Part model, mm, in its own coordinate system. A direction names the side the tool comes from. Give positions to 0.01 mm unless a question says otherwise; leave off trailing zeros. Order: outer loops, then holes, each group sorted by start corner. A loop starts at its lowest first (then second) coordinate and runs counter-clockwise, first axis right, second up. Notation, with made-up numbers: M 36.25,-8 L 81.25,-8 A21 cw 81.25,11 Z; hole C 57,47.25 d8. An arc over 180 degrees is marked long. Return JSON: item names as keys, results as strings.
from build123d import *

# Parameters (mm, degrees)
F0_W   = 1.27
F0_H   = 1.27
F0_W_2 = 3.81
F0_H_2 = 3.5783256781


with BuildPart() as f1:
    # F0 (on Front) → F1 (revolve)
    with BuildSketch(Plane.XZ):
        with BuildLine():
            Line((-12.7, 0), (0, 0))
            add(Edge.make_bspline(
                [(0, 0), (7.4514020234, 3.331559943), (-2.5339151704, 7.6260847131), (-2.54, 12.7)],
                knots=[0, 0, 0, 0, 12.9515095645, 12.9515095645, 12.9515095645, 12.9515095645], degree=3))
            Line((-2.54, 12.7), (-12.7, 12.7))
            Line((-12.7, 12.7), (-12.7, 0))
        make_face()
        with BuildLine():
            Line((-12.7, 12.7), (-2.54, 12.7))
            add(Edge.make_bspline(
                [(-2.54, 12.7), (4.5093661174, 26.4475625008), (-14.613872394, 38.6360026896), (-5.08, 50.8)],
                knots=[0, 0, 0, 0, 38.1845728011, 38.1845728011, 38.1845728011, 38.1845728011], degree=3))
            Line((-5.08, 50.8), (-12.7, 50.8))
            Line((-12.7, 50.8), (-12.7, 12.7))
        make_face()
        with BuildLine():
            Line((-12.7, 50.8), (-5.08, 50.8))
            add(Edge.make_bspline(
                [(-5.08, 50.8), (-3.208857961, 50.9595312178), (-3.3491132781, 53.203612566), (-5.08, 53.34)],
                knots=[0, 0, 0, 0, 2.54, 2.54, 2.54, 2.54], degree=3))
            Line((-5.08, 53.34), (-9.7673060372, 53.34))
            Line((-9.7673060372, 53.34), (-11.43, 53.34))
            Line((-11.43, 53.34), (-12.7, 53.34))
            Line((-12.7, 53.34), (-12.7, 50.8))
        make_face()
        with BuildLine():
            Line((-9.7673060372, 53.34), (-5.08, 53.34))
            Line((-5.08, 53.34), (-2.0844770548, 59.69))
            add(Edge.make_bspline(
                [(-11.43, 53.5471198024), (-8.0565585685, 54.6403665691), (-5.5479568491, 59.69), (-2.0844770548, 59.69)],
                knots=[1.3390316874, 1.3390316874, 1.3390316874, 1.3390316874, 12.3697949619, 12.3697949619, 12.3697949619, 12.3697949619], degree=3))
            Line((-11.43, 53.5471198024), (-11.43, 53.34))
            Line((-11.43, 53.34), (-9.7673060372, 53.34))
        make_face()
        with BuildLine():
            add(Edge.make_bspline(
                [(-12.7, 53.34), (-12.2617526092, 53.34), (-11.8395042981, 53.4144098506), (-11.43, 53.5471198024)],
                knots=[0, 0, 0, 0, 1.3390316874, 1.3390316874, 1.3390316874, 1.3390316874], degree=3))
            Line((-12.7, 53.34), (-11.43, 53.34))
            Line((-11.43, 53.34), (-11.43, 53.5471198024))
        make_face()
        with BuildLine():
            Line((-12.7, 61.1916743219), (-12.7, 53.34))
            add(Edge.make_bspline(
                [(-12.7, 53.34), (-12.2617526092, 53.34), (-11.8395042981, 53.4144098506), (-11.43, 53.5471198024)],
                knots=[0, 0, 0, 0, 1.3390316874, 1.3390316874, 1.3390316874, 1.3390316874], degree=3))
            Line((-11.43, 53.5471198024), (-11.43, 61.1916743219))
            Line((-11.43, 61.1916743219), (-12.7, 61.1916743219))
        make_face()
        with Locations((-12.065, 61.8266743219)):
            Rectangle(F0_W, F0_H)
        with Locations((-9.525, 61.8266743219)):
            Rectangle(F0_W_2, F0_H)
        with Locations((-12.065, 64.2508371609)):
            Rectangle(F0_W, F0_H_2)
    revolve(axis=Axis((-12.7, 0, 25.4), (0, 0, 1)))


with BuildPart() as f4:
    # F3 (on Front) → F4 (revolve)
    with BuildSketch(Plane.XZ):
        Polygon((-1.27, 83.82), (-1.7199835438, 78.9296406197), (0, 78.9296406197), (0, 83.82), align=None)
        Polygon((-4.4343151529, 77.1516406197), (-1.8835851687, 77.1516406197), (-1.7199835438, 78.9296406197), (-4.270713528, 78.9296406197), align=None)
        with BuildLine():
            Line((-15.5575, 0), (0, 0))
            Line((0, 0), (0, 55.88))
            Line((0, 55.88), (-5.08, 55.88))
            add(Edge.make_bspline(
                [(-15.5575, 7.62), (-12.4826701358, 22.7640494704), (-5.5103190243, 35.0550673902), (-5.08, 55.88)],
                knots=[0, 0, 0, 0, 49.3842647637, 49.3842647637, 49.3842647637, 49.3842647637], degree=3))
            Line((-15.5575, 7.62), (-15.5575, 5.08))
            ThreePointArc((-15.5575, 5.08), (-14.6594743879, 4.7080256121), (-14.2875, 3.81))
            ThreePointArc((-14.2875, 3.81), (-14.6594743879, 2.9119743879), (-15.5575, 2.54))
            Line((-15.5575, 2.54), (-15.5575, 0))
        make_face()
        Polygon((-5.08, 55.88), (0, 55.88), (0, 70.0178143454), (-2.54, 70.0178143454), (-2.4315444093, 71.1964948159), (-11.3960751224, 62.1141322649), align=None)
        Polygon((-2.54, 70.0178143454), (0, 70.0178143454), (0, 73.66), (-2.4315444093, 71.1964948159), align=None)
        Polygon((-2.4315444093, 71.1964948159), (0, 73.66), (0, 77.1516406197), (-1.8835851687, 77.1516406197), align=None)
        Polygon((-1.8835851687, 77.1516406197), (0, 77.1516406197), (0, 78.2914757729), (0, 78.9296406197), (-1.7199835438, 78.9296406197), align=None)
    revolve(axis=Axis((0, 0, 27.94), (0, 0, 1)))


solid = f4.part
Q1. Probe line 1 along Y through (x, z) = (4.5, 55); line 2 along Y through (x, z) = (0.5, 6.5); line 3 along X through (y, z) = (-10, 16.5). List the from-to ranges inside material, lowest first.
Established:
{"line 1": "y = -2.4 to 2.4", "line 2": "y = -15.55 to 15.55", "line 3": "x = -8.79 to 8.79"}
Q2. 3-axis set-ups, long thin cutter, end or side, ignore diameter. For faces 4 (the conical face through (0.865, 3.894, 69.619)), 5 (the conical face through (1.2, 0.9, 81.3)): which of +Z, -Z, +X, -X, +Y, -Y reach the whole face in a straight line?
Established:
{"face 4": "none", "face 5": "+Z"}
Q3. Two-plate mould, pull along Z, no slides. Class faces 1 (the flat face through (2, 0, 78.93)), 2 (the cylindrical face through (3.37, 15.19, 6.33)), 3 (the flat face through (-1, 2, 77.152)): +Z half, -Z half, draft (parallel to the pull), parting line (faces both ways), or undercut.
Established:
{"face 1": "+Z half", "face 2": "draft", "face 3": "undercut"}
Q4. Pin check, flat tips, straight feed: pin 1 (4 mm diameter, centred on x = -2.5, z = 23, fed in from +Y); pin 2 (1 mm diameter, centred on x = -1.5, z = 58.5, fed in from -Y); pin 3 (10 mm diameter, centred on y = 7.5, z = 47, fed in from +X). Stop position of each tip, or through.
Established:
{"pin 1": "stops at y = 11.78", "pin 2": "stops at y = -8.11", "pin 3": "stops at x = 5.2"}
Q5. Band-saw the part on A-A (z = 64). Give the cut face in (x, y).
Established:
{"outline": "C 0,0 d19.07"}
